Here's how the part is built. I have some questions about the finished solid (model axes, mm). A direction names the side the tool comes from. Give positions to 0.01 mm unless a question says otherwise; leave off trailing zeros. Loops run counter-clockwise (first coordinate to the right, second up) from the corner with the lowest first, then second, coordinate; pieces in that order, holes last.
Q1. We'd pull the mould along X, two halves only. Please class faces 1 (the face through (-1, -50.8, -16)), 2 (the face through (-30.235, -24.418, -23.183)), 3 (the face through (-12.295, -25.112, 7.231)), 4 (the face through (12.295, -25.112, -7.231)): +X half, -X half, draft (parallel to the pull), parting line (faces both ways), or undercut.
Q2. Will these pins go through, and if not, where does the flat tip stop? P1, Ø12, axis at y = -12.5, z = -8.5, coming from the -X side; P2, Ø6, axis at x = -25, y = -6, coming from the +Z side; P3, Ø3, axis at x = -6, y = -31.5, coming from the +Z side.
Q3. I need wall thicknesses on line 1 (Z direction, x = -1, y = -12); line 2 (Z direction, x = -8, y = -32.5); line 3 (X direction, y = -13.5, z = 3). Which ranges of each line are inside material? Lowest first, please.
Q4. If we section it at B-B (x = 0): Please give me the cut outline in (y, z).
Q5. If we section it at A-A (y = -6): Please give me the cut outline in (x, z).
Q6. For faces 5 (the face through (-12.75, -50.44, 7.21)), 6 (the face through (16.4, 0, 0.5)), 7 (the face through (0, -25, -14.263)), which set-ups out of +Z, -Z, +X, -X, +Y, -Y let a thin tool reach every point of the face, with its end or its side?
from build123d import *

# Parameters (mm, degrees)
F0_R     = 38.1
F1_DEPTH = 50.8
F3_DEPTH = 50.801
F4_R     = 1.27


with BuildPart() as f1:
    # F0 (on Front) → F1 (new body)
    with BuildSketch(Plane.XZ):
        Circle(F0_R)
    extrude(amount=F1_DEPTH)

    # F2 (on face) → F3 (cut, through all)
    with BuildSketch(Plane.XZ.offset(50.8)):
        Polygon((-8.2347917144, -14.263077639), (8.2347917144, -14.263077639), (16.4695834287, 0), (8.2347917144, 14.263077639), (-8.2347917144, 14.263077639), (-16.4695834287, 0), align=None)
    extrude(amount=-F3_DEPTH, mode=Mode.SUBTRACT)

    # F4
    f4_edges = [f1.edges().sort_by_distance(p)[0] for p in [
        (-38.1, -50.8, 0),
        (0, -50.8, -14.263078),
        (12.352188, -50.8, -7.131539),
        (12.352188, -50.8, 7.131539),
        (0, -50.8, 14.263078),
        (-12.352188, -50.8, 7.131539),
        (-12.352188, -50.8, -7.131539),
    ]]
    fillet(f4_edges, radius=F4_R)


solid = f1.part
Check sheet entries:
1. face 1: draft
1. face 2: parting line
1. face 3: undercut
1. face 4: undercut
2. P1: stops at x = -38.02
2. P2: stops at z = 31.11
2. P3: stops at z = 37.83
3. line 1: z = -38.09 to -14.26, 14.26 to 38.09
3. line 2: z = -37.25 to -14.26, 14.26 to 37.25
3. line 3: x = -37.98 to -14.74, 14.74 to 37.98
4. outline: (-50.8, -36.83) arc R1.27 ccw to (-49.53, -38.1) - (0, -38.1) - (0, -14.26) - (-49.53, -14.26) arc R1.27 ccw to (-50.8, -15.53) - close; (-50.8, 15.53) arc R1.27 ccw to (-49.53, 14.26) - (0, 14.26) - (0, 38.1) - (-49.53, 38.1) arc R1.27 ccw to (-50.8, 36.83) - close
5. outline: circle Ø76.2 at (0, 0); hole (-16.47, 0) - (-8.23, -14.26) - (8.23, -14.26) - (16.47, 0) - (8.23, 14.26) - (-8.23, 14.26) - close
6. face 5: -Y
6. face 6: +Z, -Z, +X, -X, +Y
6. face 7: +Y, -Y
